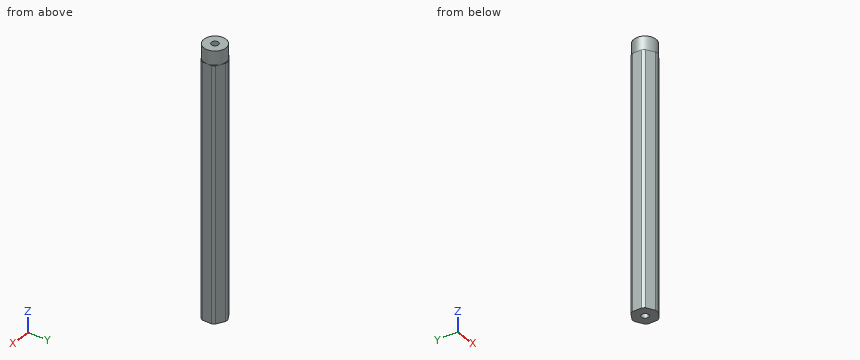
```python
from build123d import *

# Parameters (mm, degrees)
BOSS_EXTRUDE1_DEPTH    = 72.23125
SKETCH2_R              = 6.35
SKETCH2_R_2            = 2.0193
BOSS_EXTRUDE2_DEPTH    = 7.9375
F_10_32_TAPPED_HOLE1_D = 4.0386


with BuildPart() as part:
    # Sketch1 → Boss-Extrude1 (new, symmetric)
    with BuildSketch(Plane.XY):
        with BuildLine():
            ThreePointArc((0.93173274, 6.79441227), (0, 6.858), (-0.93173274, 6.79441227))
            Line((-0.93173274, 6.79441227), (-5.41826726, 4.204110358))
            ThreePointArc((-5.41826726, 4.204110358), (-5.939202219, 3.429), (-6.35, 2.590301913))
            Line((-6.35, 2.590301913), (-6.35, -2.590301913))
            ThreePointArc((-6.35, -2.590301913), (-5.939202219, -3.429), (-5.41826726, -4.204110358))
            Line((-5.41826726, -4.204110358), (-0.93173274, -6.79441227))
            ThreePointArc((-0.93173274, -6.79441227), (0, -6.858), (0.93173274, -6.79441227))
            Line((0.93173274, -6.79441227), (5.41826726, -4.204110358))
            ThreePointArc((5.41826726, -4.204110358), (5.939202219, -3.429), (6.35, -2.590301913))
            Line((6.35, -2.590301913), (6.35, 2.590301913))
            ThreePointArc((6.35, 2.590301913), (5.939202219, 3.429), (5.41826726, 4.204110358))
            Line((5.41826726, 4.204110358), (0.93173274, 6.79441227))
        make_face()
    extrude(amount=BOSS_EXTRUDE1_DEPTH, both=True)

    # Sketch2 → Boss-Extrude2 (add)
    with BuildSketch(Plane.XY.offset(72.23125)):
        Circle(SKETCH2_R)
        Circle(SKETCH2_R_2, mode=Mode.SUBTRACT)
    extrude(amount=BOSS_EXTRUDE2_DEPTH)

    # #10-32 Tapped Hole1 (through all)
    with Locations(Plane(origin=(0, 0, -72.23125), x_dir=(-1, 0, 0), z_dir=(0, 0, -1))):
        with Locations((0, 0)):
            Hole(F_10_32_TAPPED_HOLE1_D / 2)


solid = part.part
```
Part model, mm, in its own coordinate system. Round coordinates to 2 decimals unless told otherwise and drop trailing zeros. Write each loop counter-clockwise with the first axis right and the second up, starting at its lowest first coordinate (ties: lowest second). Pieces come first, ordered by that corner, then holes.
Item 1: Cut at A-A, the plane z = -42. Give the cut face in (x, y), plus the area to 3 significant figures.
Results:
outline: (-6.35, -2.59) arc R6.86 ccw to (-5.42, -4.2) - (-0.93, -6.79) arc R6.86 ccw to (0.93, -6.79) - (5.42, -4.2) arc R6.86 ccw to (6.35, -2.59) - (6.35, 2.59) arc R6.86 ccw to (5.42, 4.2) - (0.93, 6.79) arc R6.86 ccw to (-0.93, 6.79) - (-5.42, 4.2) arc R6.86 ccw to (-6.35, 2.59) - close; hole circle Ø4.04 at (0, 0)
area: 124 mm2
Item 2: Probe L1, parallel to Y at x = -0.25, z = 49.5; L2, parallel to X at y = 0.5, z = 36; L3, parallel to X at y = 1.5, z = -55. List the from-to ranges inside material, lowest first.
Results:
L1: y = -6.85 to -2, 2 to 6.85
L2: x = -6.35 to -1.96, 1.96 to 6.35
L3: x = -6.35 to -1.35, 1.35 to 6.35
Item 3: Drop flat-ended pins along their axis: pin 1 Ø1.6 at (x, y) = (-5.5, 3.5) entering from +Z; pin 2 Ø1.5 at (x, z) = (3.5, -37) entering from -Y; pin 3 Ø3 at (x, z) = (2, -11) entering from +Y; pin 4 Ø1 at (x, z) = (4.5, -11.5) entering from +Y. Give the stop position or say it passes through.
Results:
pin 1: stops at z = 80.17
pin 2: stops at y = -5.74
pin 3: stops at y = 6.84
pin 4: stops at y = 5.02
